from build123d import *

# Parameters (mm, degrees)
F0_W     = 50.8
F0_H     = 6.35
F1_DEPTH = 88.9
F2_R     = 2.6162
F2_R_2   = 2.5
F3_DEPTH = 6.351
F4_R     = 3.175


with BuildPart() as f1:
    # F0 (on Front) → F1 (new body)
    with BuildSketch(Plane.XZ):
        Rectangle(F0_W, F0_H)
    extrude(amount=F1_DEPTH)

    # F2 (on face) → F3 (cut, through all)
    with BuildSketch(Plane.XY.offset(3.175)):
        with Locations((0, -82.55)):
            Circle(F2_R)
        with Locations((0, -6.35)):
            Circle(F2_R)
        with Locations((-19.05, -82.55)):
            Circle(F2_R)
        with Locations((19.05, -82.55)):
            Circle(F2_R)
        with Locations((19.05, -6.35)):
            Circle(F2_R)
        with Locations((-19.05, -6.35)):
            Circle(F2_R)
        with Locations((-15, -60.45)):
            Circle(F2_R_2)
        with Locations((15, -60.45)):
            Circle(F2_R_2)
        with Locations((15, -28.45)):
            Circle(F2_R_2)
        with Locations((-15, -28.45)):
            Circle(F2_R_2)
    extrude(amount=-F3_DEPTH, mode=Mode.SUBTRACT)

    # F4
    f4_edges = [f1.edges().sort_by_distance(p)[0] for p in [
        (0, 0, 3.175),
        (0, -88.9, 3.175),
    ]]
    fillet(f4_edges, radius=F4_R)


solid = f1.part
The listing builds one solid part. Answer for the finished solid, in the listing's coordinates (mm). Round coordinates to 2 decimals unless told otherwise and drop trailing zeros. Write each loop counter-clockwise with the first axis right and the second up, starting at its lowest first coordinate (ties: lowest second). Pieces come first, ordered by that corner, then holes. Notation, with made-up numbers: (-18.75, 47) - (31.25, 47) arc R23 ccw to (31.25, 68) - close; hole circle Ø5 at (12.5, -4). An arc over 180 degrees is marked (long way). Use a Markdown table: item, result. Add a question column.
1. The part is cut by section D-D (y = -28.45). Write down the section's boundary in (x, z) (3 decimals).
2. Consider line 1 (Y direction, x = -19.05, z = -1.25); line 2 (X direction, y = -60, z = 1); line 3 (Y direction, x = 0, z = 1.5). Determine where each line is inside the solid, lowest interval first.
3. The part is cut by section B-B (y = -6.35). Write down the section's boundary in (x, z) (3 decimals).
4. The part is cut by section C-C (z = -2.25). Give the number of separate pieces and of enclosed holes in the cut face, and give its area (3 significant figures).
5. For a pull along X with two mould halves and no side action, classify faces 1 (the face through (0, -44, -3.175)), 2 (the face through (-15.5, -30.9, 0)), 3 (the face through (25.4, -44, 0)) as +X half, -X half, draft (parallel to the pull), parting line (faces both ways), or undercut.
6. The part is cut by section A-A (x = -19.05). Write down the section's boundary in (y, z) (3 decimals), and give its area (3 significant figures).
Reported:
| question | item | result |
|---|---|---|
| 1 | outline | (-25.4, -3.175) - (-17.5, -3.175) - (-17.5, 3.175) - (-25.4, 3.175) - close; (-12.5, -3.175) - (12.5, -3.175) - (12.5, 3.175) - (-12.5, 3.175) - close; (17.5, -3.175) - (25.4, -3.175) - (25.4, 3.175) - (17.5, 3.175) - close |
| 2 | line 1 | -88.9 to -85.17, -79.93 to -8.97, -3.73 to 0 |
| 2 | line 2 | -25.4 to -17.46, -12.54 to 12.54, 17.46 to 25.4 |
| 2 | line 3 | -88.52 to -85.17, -79.93 to -8.97, -3.73 to -0.38 |
| 3 | outline | (-25.4, -3.175) - (-21.666, -3.175) - (-21.666, 3.175) - (-25.4, 3.175) - close; (-16.434, -3.175) - (-2.616, -3.175) - (-2.616, 3.175) - (-16.434, 3.175) - close; (2.616, -3.175) - (16.434, -3.175) - (16.434, 3.175) - (2.616, 3.175) - close; (21.666, -3.175) - (25.4, -3.175) - (25.4, 3.175) - (21.666, 3.175) - close |
| 4 | separate pieces | 1 |
| 4 | enclosed holes | 10 |
| 4 | area | 4,310 mm^2 |
| 5 | face 1 | draft |
| 5 | face 2 | undercut |
| 5 | face 3 | +X half |
| 6 | outline | (-88.9, -3.175) - (-85.166, -3.175) - (-85.166, 3.175) - (-85.725, 3.175) arc R3.175 ccw to (-88.9, 0) - close; (-79.934, -3.175) - (-8.966, -3.175) - (-8.966, 3.175) - (-79.934, 3.175) - close; (-3.734, -3.175) - (0, -3.175) - (0, 0) arc R3.175 ccw to (-3.175, 3.175) - (-3.734, 3.175) - close |
| 6 | area | 494 mm^2 |
